```python
from build123d import *

# Parameters (mm, degrees)
PAD_DEPTH            = 1.9
THICKNESS_T          = 0.7
SKETCH001_W          = 18
SKETCH001_H          = 3
POCKET_DEPTH         = 1
POCKET_DEPTH_BACK    = 5
POCKET001_START      = -0.6
SKETCH002_W          = 49.648089
SKETCH002_H          = 49.770681
POCKET001_DEPTH      = 1.4
SKETCH011_W          = 18
SKETCH011_H          = 0.8
POCKET005_DEPTH      = 2.5
SKETCH035_W          = 17.144912
SKETCH035_H          = 0.2
SKETCH035_W_2        = 0.2
SKETCH035_H_2        = 13.969912
POCKET015_DEPTH      = 5
BODY_PLACEMENT_ANGLE = 270


with BuildPart() as part:
    # Sketch → Pad (new body)
    with BuildSketch(Plane.XY):
        with BuildLine():
            Line((-15.185, 13.864998), (-15.185, -13.864986))
            ThreePointArc((-15.185, -13.864986), (-13.720534, -17.40052), (-10.185, -18.864986))
            Line((-10.185, -18.864986), (10.184984, -18.864986))
            ThreePointArc((10.184984, -18.864986), (13.720524, -17.400521), (15.185, -13.864986))
            Line((15.185, 13.864998), (15.185, -13.864986))
            ThreePointArc((15.185, 13.864998), (13.720535, 17.400537), (10.185, 18.865014))
            Line((-10.184984, 18.865014), (10.185, 18.865014))
            ThreePointArc((-10.184984, 18.865014), (-13.720529, 17.400543), (-15.185, 13.864998))
        make_face()
    extrude(amount=PAD_DEPTH)

    # Thickness
    thickness_openings = [part.faces().sort_by_distance(p)[0] for p in [
        (0, 1.3e-05, 1.9),
    ]]
    offset(amount=THICKNESS_T, openings=thickness_openings, kind=Kind.INTERSECTION)

    # Sketch001 → Pocket (cut, two sides)
    with BuildSketch(Plane.XY) as pocket_sk:
        with Locations((0, 17.865014)):
            Rectangle(SKETCH001_W, SKETCH001_H)
    extrude(amount=POCKET_DEPTH, mode=Mode.SUBTRACT)
    extrude(pocket_sk.sketch, amount=-POCKET_DEPTH_BACK, mode=Mode.SUBTRACT)

    # Sketch002 → Pocket001 (cut)
    with BuildSketch(Plane.XY.offset(POCKET001_START)):
        with Locations((-0.449389, 1.150265)):
            Rectangle(SKETCH002_W, SKETCH002_H)
    extrude(amount=-POCKET001_DEPTH, mode=Mode.SUBTRACT)

    # Sketch011 → Pocket005 (cut, symmetric)
    with BuildSketch(Plane.XY):
        with Locations((0, 19.265014)):
            Rectangle(SKETCH011_W, SKETCH011_H)
    extrude(amount=POCKET005_DEPTH, both=True, mode=Mode.SUBTRACT)

    # Sketch035 → Pocket015 (cut)
    with BuildSketch(Plane.XY):
        with Locations((-4.004159, 2.3314)):
            Rectangle(SKETCH035_W, SKETCH035_H)
        with Locations((7.573341, -7.6586)):
            Rectangle(SKETCH035_W_2, SKETCH035_H_2)
    extrude(amount=-POCKET015_DEPTH, mode=Mode.SUBTRACT)


with BuildPart() as part_1:
    # Body placement: moved
    add(part.part.moved(Location((0.2, 12.9, 10))).rotate(Axis((0.2, 12.9, 10), (0, 0, 1)), BODY_PLACEMENT_ANGLE))


solid = part_1.part
```
Part model, mm, in its own coordinate system. A direction names the side the tool comes from. Round coordinates to 2 decimals unless told otherwise and drop trailing zeros. Loops run counter-clockwise (first coordinate to the right, second up) from the corner with the lowest first, then second, coordinate; pieces in that order, holes last. Notation, with made-up numbers: (-5, -35) -> (6, -35) arc R13 ccw to (6, -31) -> close; hole circle Ø9 at (-38, 66.25). An arc over 180 degrees is marked (long way). Use CSV: the item, a comma, the result in double quotes. Start each with the question number.
1) Pull direction X, two halves, no side cores. Call faces 4 (the cylindrical face through (18.05, -1.36, 10.63)), 5 (the cylindrical face through (-17.16, 26.66, 10.94)), 6 (the flat face through (0, 28.785, 11)): +X half, -X half, draft (parallel to the pull), parting line (faces both ways), or undercut.
2) Cut at A-A, the plane y = 18. Write the cut outline in (x, z).
3) Drop flat-ended pins along their axis: P1, Ø1.5, axis at x = 11, y = 7, coming from the +Z side; P2, Ø0.7, axis at y = 12, z = 9.5, coming from the +X side (3 decimals); P3, Ø0.6, axis at y = 12.5, z = 11, coming from the +X side (3 decimals). Give the stop position or say it passes through.
4) Cut at D-D, the plane z = 11.2. Write the cut outline in (x, y) (3 decimals), plus the area to 3 significant figures.
5) Cut at B-B, the plane x = -10.5. Write the cut outline in (y, z) (3 decimals), plus the area to 3 significant figures.
6) Wall check: L1, parallel to X at y = 15.5, z = 9.7; L2, parallel to Y at x = -2, z = 9.8 (3 decimals); L3, parallel to Y at x = -1, z = 11.6 (3 decimals). Give the ranges that are in metal, low to high. Write a range as [from, to].
7) Cut at C-C, the plane x = 7. Write the cut outline in (y, z) (3 decimals), plus the area to 3 significant figures.
8) Which spindle directions (+Z, -Z, +X, -X, +Y, -Y) get a long thin tool onto all of the face, cutting with end or side? Do faces 1 (the flat face through (0.3, 28.3, 11.9)), 2 (the flat face through (18.9, 21.9, 9.8)), 3 (the cylindrical face through (-17.24, -0.78, 10.94)). Say none if no direction does.
Determined:
1,face 4,"+X half"
1,face 5,"undercut"
1,face 6,"draft"
2,outline,"(-19.36, 9.4) -> (2.43, 9.4) -> (2.43, 10) -> (-18.66, 10) -> (-18.66, 11.9) -> (-19.36, 11.9) -> close; (2.63, 9.4) -> (16.57, 9.4) -> (16.57, 10) -> (2.63, 10) -> close"
3,P1,"stops at z = 10"
3,P2,"stops at x = 16.565"
3,P3,"stops at x = -18.665"
4,outline,"(-19.365, 2.715) arc R5.7 ccw to (-13.665, -2.985) -> (14.065, -2.985) arc R5.7 ccw to (19.765, 2.715) -> (19.765, 3.9) -> (19.065, 3.9) -> (19.065, 2.715) arc R5 cw to (14.065, -2.285) -> (-13.665, -2.285) arc R5 cw to (-18.665, 2.715) -> (-18.665, 23.085) arc R5 cw to (-13.665, 28.085) -> (14.065, 28.085) arc R5 cw to (19.065, 23.085) -> (19.065, 21.9) -> (19.765, 21.9) -> (19.765, 23.085) arc R5.7 ccw to (14.065, 28.785) -> (-13.665, 28.785) arc R5.7 ccw to (-19.365, 23.085) -> close"
4,area,"78.3 mm2"
5,outline,"(-2.985, 9.4) -> (5.227, 9.4) -> (5.227, 10) -> (-2.285, 10) -> (-2.285, 11.9) -> (-2.985, 11.9) -> close; (5.427, 9.4) -> (28.785, 9.4) -> (28.785, 11.9) -> (28.085, 11.9) -> (28.085, 10) -> (5.427, 10) -> close"
5,area,"21.6 mm2"
6,L1,"x = [-19.36, 2.43], [2.63, 16.57]"
6,L2,"y = [-2.985, 5.227], [5.427, 28.785]"
6,L3,"y = [-2.985, -2.285], [28.085, 28.785]"
7,outline,"(-2.985, 9.4) -> (28.785, 9.4) -> (28.785, 11.9) -> (28.085, 11.9) -> (28.085, 10) -> (-2.285, 10) -> (-2.285, 11.9) -> (-2.985, 11.9) -> close"
7,area,"21.7 mm2"
8,face 1,"+Z, +X, -X, +Y, -Y"
8,face 2,"+Z, -Z, +X"
8,face 3,"+Z"
